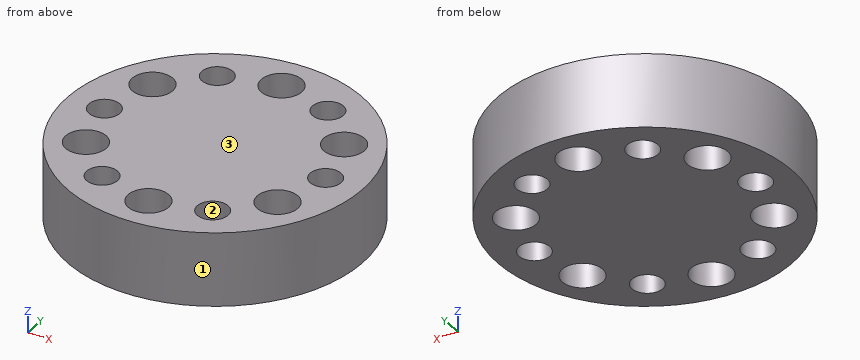
Autodesk Inventor part; units mm, degrees
ref_plane "YZ Plane" through (0, 0, 0) normal (1, 0, 0) x (0, 1, 0)
ref_plane "XZ Plane" through (0, 0, 0) normal (0, 1, 0) x (-1, 0, 0)
ref_plane "XY Plane" through (0, 0, 0) normal (0, 0, 1) x (1, 0, 0)
sketch "Esboço1" plane through (0, 0, 0) normal (0, 0, 1) x (1, 0, 0)
  circle A0 centre (0, 0) radius 40
  dimension "d0" = 80
extrude "Extrusão1" add sketch "Esboço1" along normal blind 20
sketch "Esboço2" plane through (0, 0, 20) normal (0, 0, 1) x (1, 0, 0)
  point P0 (0, 0)
  point P1 (0, 30)
  dimension "d3" = 30
hole "Furo1" at (0, 30, 20) direction (0, 0, -1) diameter 11 end through all
pattern_circular "Padrão circular1" count 6 over 360 about axis through (0, 0, 0) along (0, 0, 1) of "Furo1"
sketch "Esboço3" plane through (0, 0, 20) normal (0, 0, 1) x (1, 0, 0)
  circle A0 centre (0, 30) radius 5.5
  circle A1 centre (0, 0) radius 30 construction
  line L0 (0, 0) -> (-62.0397, 0) construction
  line L1 (0, 0) -> (-27.415, 47.4843)
  point P0 (-15, 25.9808)
  dimension "d14" = 60
hole "Furo2" at (-15, 25.9808, 20) direction (0, 0, -1) diameter 8.376 end through all
pattern_circular "Padrão circular2" count 6 over 360 about axis through (0, 0, 0) along (0, 0, 1) of "Furo2"
properties part number "3D Model"
Geometry check sheet. Reference: the model listing, model coordinates, mm. Face numbers are marked on the shaded views. Round coordinates to 2 decimals unless told otherwise and drop trailing zeros. Order: outer loops, then holes, each group sorted by start corner. A loop starts at its lowest first (then second) coordinate and runs counter-clockwise, first axis right, second up. Notation, with made-up numbers: M 83.5,-30.5 L 109.5,-30.5 A20 ccw 109.5,-5.5 Z; hole C 74,64 d7. An arc over 180 degrees is marked long. Write item = value, one per line.
Q1. Section check C-C (y = -26.5). Enter the section's corners in (x, z), plus the area to 3 significant figures.
Answer block:
outline = M -29.96,0 L -19.16,0 L -19.16,20 L -29.96,20 Z; M -10.84,0 L -4.24,0 L -4.24,20 L -10.84,20 Z; M 4.24,0 L 10.84,0 L 10.84,20 L 4.24,20 Z; M 19.16,0 L 29.96,0 L 29.96,20 L 19.16,20 Z
area = 696 mm^2
Q2. Scan lines: line 1 (Y direction, x = 2, z = 8.5); line 2 (X direction, y = 29, z = 11.75); line 3 (Y direction, x = -15, z = 15). Record each from-to range of solid material in increasing order.
Answer block:
line_1 = -39.95 to -35.12, -24.88 to 24.88, 35.12 to 39.95
line_2 = -27.55 to -17.9, -12.1 to -5.41, 5.41 to 12.1, 17.9 to 27.55
line_3 = -37.08 to -30.17, -21.79 to 21.79, 30.17 to 37.08
Q3. Release check for a two-part mould opening along Y. For the marked faces 1, 2 and 3 record: released by +Y, released by -Y, zero draft, split by the parting line, or undercut.
Answer block:
face_1 = split by the parting line
face_2 = undercut
face_3 = zero draft
Q4. Section check B-B (x = 3.5). Enter the section's corners in (y, z), plus the area to 3 significant figures.
Answer block:
outline = M -39.85,0 L -34.24,0 L -34.24,20 L -39.85,20 Z; M -25.76,0 L 25.76,0 L 25.76,20 L -25.76,20 Z; M 34.24,0 L 39.85,0 L 39.85,20 L 34.24,20 Z
area = 1,250 mm^2
Q5. Section check A-A (y = 0). Enter the section's corners in (x, z), plus the area to 3 significant figures.
Answer block:
outline = M -40,0 L -34.19,0 L -34.19,20 L -40,20 Z; M -25.81,0 L 25.81,0 L 25.81,20 L -25.81,20 Z; M 34.19,0 L 40,0 L 40,20 L 34.19,20 Z
area = 1,260 mm^2
Q6. Depth check by flat-ended pin: pin 1 Ø3 at (y, z) = (22.5, 11) entering from -X; pin 2 Ø8 at (y, z) = (-13.5, 5.5) entering from +X; pin 3 Ø4 at (x, z) = (14.5, 2.5) entering from +Y; pin 4 Ø5 at (x, y) = (15, 25.98) entering from +Z. Enter the tip coordinate at first touch or a pass-through.
Answer block:
pin_1 = -34.04
pin_2 = 38.86
pin_3 = 38
pin_4 = through
Q7. Section check D-D (z = 1.75). Give the number of separate pieces and of enclosed holes in the cut face, plus the area to 3 significant figures.
Answer block:
separate_pieces = 1
enclosed_holes = 12
area = 4,130 mm^2
